Can you work these out from the model? Positions are in its coordinate system, mm. A direction names the side the tool comes from. Round coordinates to 2 decimals unless told otherwise and drop trailing zeros. Order: outer loops, then holes, each group sorted by start corner. A loop starts at its lowest first (then second) coordinate and runs counter-clockwise, first axis right, second up. Notation, with made-up numbers: (-25, -27.75) -> (29, -27.75) arc R17 cw to (29, -3.75) -> close; hole circle Ø2 at (37.5, -24). An arc over 180 degrees is marked (long way). One line per item, written item: value.
```python
from build123d import *

# Parameters (mm, degrees)
SKETCH_1_R          = 1.7
SKETCH_1_R_2        = 1.5
SKETCH_1_R_3        = 2
SKETCH_1_R_4        = 5.1
SKETCH_1_R_5        = 1.65
EXTRUDE_1_DEPTH     = 3
SKETCH_3_R          = 1
CUT_EXTRUDE_3_DEPTH = 124.273070863
CUT_EXTRUDE_4_DEPTH = 124.273070863
EXTRUDE_START       = -3
EXTRUDE_1_2_DEPTH   = 3
EXTRUDE_2_DEPTH     = 3
FILLET_4_R          = 1
FILLET_6_R          = 5
FILLET_7_R          = 3


# Read off the part's stored shape, not the designer's step: 拉伸-薄壁1
with BuildPart() as part:
    # 草图1 → Extrude 1 (new body)
    with BuildSketch(Plane(origin=(0, 0, 0), x_dir=(1, 0, 0), z_dir=(0, 1, 0))):
        with BuildLine():
            Line((-51.003122908, 26.550545261), (-40.35899291, 21.009561902))
            ThreePointArc((-40.35899291, 21.009561902), (0, -45.5), (40.35899291, 21.009561902))
            Line((40.35899291, 21.009561902), (51.003122908, 26.550545261))
            ThreePointArc((51.003122908, 26.550545261), (57.123657521, 6.567933576), (55.697982668, -14.282322175))
            Line((55.697982668, -14.282322175), (35, -95))
            Line((35, -95), (35, -105))
            Line((35, -105), (20, -105))
            Line((20, -105), (20, -109))
            Line((20, -109), (-20, -109))
            Line((-20, -109), (-20, -105))
            Line((-20, -105), (-35, -105))
            Line((-35, -105), (-35, -95))
            Line((-35, -95), (-55.697982668, -14.282322175))
            ThreePointArc((-55.697982668, -14.282322175), (-57.123657521, 6.567933576), (-51.003122908, 26.550545261))
        make_face()
        with Locations(Location((8.091010553, -58.777423797, 0), (0, 0, 270))):
            Circle(SKETCH_1_R, mode=Mode.SUBTRACT)
        with Locations(Location((31.583326073, -50.226920214, 0), (0, 0, 270))):
            Circle(SKETCH_1_R, mode=Mode.SUBTRACT)
        with Locations(Location((-31, -100, 0), (0, 0, 270))):
            Circle(SKETCH_1_R_2, mode=Mode.SUBTRACT)
        with Locations(Location((31, -100, 0), (0, 0, 90))):
            Circle(SKETCH_1_R_2, mode=Mode.SUBTRACT)
        with Locations(Location((-37.123106012, -37.123106012, 0), (0, 0, 270))):
            Circle(SKETCH_1_R_3, mode=Mode.SUBTRACT)
        with Locations(Location((-52.5, 0, 0), (0, 0, 270))):
            Circle(SKETCH_1_R_3, mode=Mode.SUBTRACT)
        with Locations(Location((52.5, 0, 0), (0, 0, 270))):
            Circle(SKETCH_1_R_3, mode=Mode.SUBTRACT)
        with Locations(Location((37.123106012, -37.123106012, 0), (0, 0, 270))):
            Circle(SKETCH_1_R_3, mode=Mode.SUBTRACT)
        with Locations(Location((19.837168313, -54.502172006, 0), (0, 0, 270))):
            Circle(SKETCH_1_R_4, mode=Mode.SUBTRACT)
        with Locations(Location((32.925309654, -89, 0), (0, 0, 270))):
            Circle(SKETCH_1_R_5, mode=Mode.SUBTRACT)
        with Locations(Location((36.65113283, -74.470091478, 0), (0, 0, 270))):
            Circle(SKETCH_1_R_5, mode=Mode.SUBTRACT)
    extrude(amount=EXTRUDE_1_DEPTH)

    # 草图3 → 切除-拉伸3 (cut, through all)
    with BuildSketch(Plane(origin=(0, 3, 0), x_dir=(1, 0, 0), z_dir=(0, 1, 0))):
        with Locations((-21, -105)):
            Circle(SKETCH_3_R)
        with Locations((21, -105)):
            Circle(SKETCH_3_R)
    extrude(amount=-CUT_EXTRUDE_3_DEPTH, mode=Mode.SUBTRACT)

    # 草图4 → 切除-拉伸4 (cut, through all)
    with BuildSketch(Plane(origin=(0, 3, 0), x_dir=(1, 0, 0), z_dir=(0, 1, 0))):
        with BuildLine():
            Line((-30.440624747, -80.572934593), (-12.021970306, -56.229193752))
            ThreePointArc((-12.021970306, -56.229193752), (-23.121395009, -52.646472748), (-33.269507662, -46.897653033))
            ThreePointArc((-33.269507662, -46.897653033), (-32.970979927, -55.81081258), (-34.539030241, -64.590035219))
            Line((-34.539030241, -64.590035219), (-30.440624747, -80.572934593))
        make_face()
        Polygon((19.433888905, -66.025448201), (34.930515062, -63.063328668), (30.440624747, -80.572934593), align=None)
        with BuildLine():
            Line((28.536143905, -88), (0, -103))
            Line((0, -103), (-28.536143905, -88))
            Line((-28.536143905, -88), (-12.86067095, -67.281893127))
            ThreePointArc((-12.86067095, -67.281893127), (0, -68.5), (12.86067095, -67.281893127))
            Line((12.86067095, -67.281893127), (28.536143905, -88))
        make_face()
        with BuildLine():
            Line((-42.861253018, -64.342805115), (-55.697982668, -14.282322175))
            ThreePointArc((-55.697982668, -14.282322175), (-52.242961211, -24.01922155), (-47.101242547, -32.98064509))
            ThreePointArc((-47.101242547, -32.98064509), (-41.173018347, -48.146873673), (-42.861253018, -64.342805115))
        make_face()
    extrude(amount=-CUT_EXTRUDE_4_DEPTH, mode=Mode.SUBTRACT)

    # Extrude 1 2 outline → Extrude 1 2 (add)
    with BuildSketch(Plane(origin=(0, 3, 0), x_dir=(1, 0, 0), z_dir=(0, 1, 0)).offset(EXTRUDE_START)):
        with BuildLine():
            Line((21.778618406, -79.068649994), (18.835174857, -75.178331775))
            Line((18.835174857, -75.178331775), (3.50933235, -68.410047409))
            ThreePointArc((3.50933235, -68.410047409), (0, -68.5), (-3.50933235, -68.410047409))
            Line((-3.50933235, -68.410047409), (-18.835174857, -75.178331775))
            Line((-18.835174857, -75.178331775), (-21.778618406, -79.068649994))
            Line((-21.778618406, -79.068649994), (-16.234523365, -94.466336472))
            Line((-16.234523365, -94.466336472), (-11.414457562, -97))
            Line((-11.414457562, -97), (11.414457562, -97))
            Line((11.414457562, -97), (16.234523365, -94.466336472))
            Line((16.234523365, -94.466336472), (21.778618406, -79.068649994))
        make_face()
        Polygon((-12.743110853, -89.403790429), (-16.300181473, -79.524692438), (-4.850437176, -74.468192262), align=None, mode=Mode.SUBTRACT)
        Polygon((0, -75.991095057), (8.459859541, -92), (-8.459859541, -92), align=None, mode=Mode.SUBTRACT)
        Polygon((4.850437176, -74.468192262), (16.300181473, -79.524692438), (12.743110853, -89.403790429), align=None, mode=Mode.SUBTRACT)
    extrude(amount=EXTRUDE_1_2_DEPTH)

    # 草图5<3> → 拉伸-薄壁2 (add)
    with BuildSketch(Plane(origin=(0, 3, 0), x_dir=(1, 0, 0), z_dir=(0, 1, 0))):
        Polygon((-35.554014882, -67.633687886), (-11.151745265, -58.572846537), (-12.892195346, -53.885540966), (-37.294464963, -62.946382315), align=None)
    extrude(amount=-EXTRUDE_2_DEPTH)

    # 圆角4
    fillet_4_edges = [part.edges().sort_by_distance(p)[0] for p in [
        (30.440624747, 1.5, 80.572934593),
        (19.433888905, 1.5, 66.025448201),
        (34.930515062, 1.5, 63.063328668),
        (-12.86067095, 1.5, 67.281893127),
        (12.86067095, 1.5, 67.281893127),
        (28.536143905, 1.5, 88),
        (0, 1.5, 103),
        (-28.536143905, 1.5, 88),
        (-30.440624747, 1.5, 80.572934593),
        (-33.269507662, 1.5, 46.897653033),
        (-21.778618406, 1.5, 79.068649994),
        (-18.835174857, 1.5, 75.178331775),
        (-11.414457562, 1.5, 97),
        (16.234523365, 1.5, 94.466336472),
        (18.835174857, 1.5, 75.178331775),
        (3.50933235, 1.5, 68.410047409),
        (21.778618406, 1.5, 79.068649994),
        (11.414457562, 1.5, 97),
        (-3.50933235, 1.5, 68.410047409),
        (-16.234523365, 1.5, 94.466336472),
        (-16.300181473, 1.5, 79.524692438),
        (4.850437176, 1.5, 74.468192262),
        (16.300181473, 1.5, 79.524692438),
        (12.743110853, 1.5, 89.403790429),
        (-4.850437176, 1.5, 74.468192262),
        (-12.743110853, 1.5, 89.403790429),
        (8.459859541, 1.5, 92),
        (-8.459859541, 1.5, 92),
        (0, 1.5, 75.991095057),
        (35, 1.5, 105),
        (20, 1.5, 109),
        (-20, 1.5, 109),
        (-35, 1.5, 105),
        (-14.827987759, 1.5, 59.937877353),
        (-16.285565355, 1.5, 55.145537998),
        (-33.79999967, 1.5, 61.648847449),
        (-33.914652527, 1.5, 67.024973924),
    ]]
    fillet(fillet_4_edges, radius=FILLET_4_R)

    # 圆角6
    fillet_6_edges = [part.edges().sort_by_distance(p)[0] for p in [
        (-42.861253018, 1.5, 64.342805115),
        (-35, 1.5, 95),
        (35, 1.5, 95),
    ]]
    fillet(fillet_6_edges, radius=FILLET_6_R)

    # 圆角7
    fillet_7_edges = [part.edges().sort_by_distance(p)[0] for p in [
        (-51.003122908, 1.5, -26.550545261),
        (-40.35899291, 1.5, -21.009561902),
        (40.35899291, 1.5, -21.009561902),
        (51.003122908, 1.5, -26.550545261),
    ]]
    fillet(fillet_7_edges, radius=FILLET_7_R)


solid = part.part
```
Q1. We'd pull the mould along Z, two halves only. Please class faces 4 (the face through (-38.775, 1.479, 80.279)), 5 (the face through (-11.521, 1.479, 77.414)): released by +Z, released by -Z, zero draft, split by the parting line, or undercut.
Answers below:
face 4: released by +Z
face 5: undercut
Q2. On a 3-axis mill with a long thin cutter (end or side, diameter ignored), from which of +Z, -Z, +X, -X, +Y, -Y can I reach the whole of each face in a straight line? I mean faces 1 (the face through (-23.13, 1.52, 70.91)), 2 (the face through (-28, 1, 105)), 3 (the face through (-42.65, 1.48, 64.38)). Say none if no direction works.
Answers below:
face 1: +Y, -Y
face 2: +Z, -X, +Y, -Y
face 3: -X, +Y, -Y
Q3. Please list where these lines run through material, in increasing order: line 1 along X through (y, z) = (2.05, 0); line 2 along Z through (x, y) = (16.5, 0.45); line 3 along Z through (x, y) = (9.5, 1.4).
Answers below:
line 1: -57.5 to -54.5, -50.5 to -45.5, 45.5 to 50.5, 54.5 to 57.5
line 2: 42.4 to 50.65, 58.36 to 72.09, 73.32 to 109
line 3: 44.5 to 57.83, 59.73 to 67.84, 71.06 to 76.52, 83.27 to 109
Q4. Will this pin go through, and if not, where does the flat tip stop? pin 1 Ø0.9 at (y, z) = (2, 101) entering from -X.
Answers below:
pin 1: x = -35
Q5. I want a section at A-A on z = 0. List the corners of the cut face in (x, y) for me.
Answers below:
outline: (-57.5, 0) -> (-54.5, 0) -> (-54.5, 3) -> (-57.5, 3) -> close; (-50.5, 0) -> (-45.5, 0) -> (-45.5, 3) -> (-50.5, 3) -> close; (45.5, 0) -> (50.5, 0) -> (50.5, 3) -> (45.5, 3) -> close; (54.5, 0) -> (57.5, 0) -> (57.5, 3) -> (54.5, 3) -> close
Q6. I want a section at B-B on y = 1.3. Give the number of separate pieces and of enclosed holes in the cut face, plus the area to 3 significant figures.
Answers below:
separate pieces: 1
enclosed holes: 22
area: 5,880 mm^2
